Here's how the part is built. I have some questions about the finished solid (model axes, mm). A direction names the side the tool comes from. Round coordinates to 2 decimals unless told otherwise and drop trailing zeros. Loops run counter-clockwise (first coordinate to the right, second up) from the corner with the lowest first, then second, coordinate; pieces in that order, holes last. Notation, with made-up numbers: (20.25, -18.5) -> (41.25, -18.5) arc R13 ccw to (41.25, -5.5) -> close; hole circle Ø1 at (89, 88.5). An arc over 180 degrees is marked (long way). One line per item, written item: value. Start each with the question number.
```python
from build123d import *

# Parameters (mm, degrees)
SKETCH1_W           = 5.08
SKETCH1_H           = 203.2
BOSS_EXTRUDE1_DEPTH = 152.4
SKETCH2_W           = 88.9
SKETCH2_H           = 50.8
CUT_EXTRUDE1_DEPTH  = 5.08
SKETCH3_W           = 5.08
SKETCH3_H           = 10.16
CUT_EXTRUDE2_DEPTH  = 5.08
SKETCH5_W           = 5.08
SKETCH5_H           = 25.4
BOSS_EXTRUDE2_DEPTH = 5.08
SKETCH6_W           = 25.4
SKETCH6_H           = 5.08
SKETCH6_W_2         = 5.08
SKETCH6_H_2         = 25.4
CUT_EXTRUDE3_DEPTH  = 5.08


with BuildPart() as part:
    # Sketch1 → Boss-Extrude1 (new body)
    with BuildSketch(Plane.XY):
        with Locations((-99.06, 0)):
            Rectangle(SKETCH1_W, SKETCH1_H)
    extrude(amount=BOSS_EXTRUDE1_DEPTH)

    # Sketch2 → Cut-Extrude1 (cut)
    with BuildSketch(Plane.ZY.offset(101.6)):
        with Locations((107.95, -76.2)):
            Rectangle(SKETCH2_W, SKETCH2_H)
    extrude(amount=-CUT_EXTRUDE1_DEPTH, mode=Mode.SUBTRACT)

    # Sketch3 → Cut-Extrude2 (cut)
    with BuildSketch(Plane.XZ.offset(101.6)):
        with Locations((-99.06, 46.99)):
            Rectangle(SKETCH3_W, SKETCH3_H)
        with Locations((-99.06, 16.51)):
            Rectangle(SKETCH3_W, SKETCH3_H)
    extrude(amount=-CUT_EXTRUDE2_DEPTH, mode=Mode.SUBTRACT)

    # Sketch5 → Boss-Extrude2 (add)
    with BuildSketch(Plane(origin=(0, 0, 0), x_dir=(-1, 0, 0), z_dir=(0, 0, -1))):
        with Locations((99.06, -44.45)):
            Rectangle(SKETCH5_W, SKETCH5_H)
        with Locations((99.06, 63.5)):
            Rectangle(SKETCH5_W, SKETCH5_H)
    extrude(amount=BOSS_EXTRUDE2_DEPTH)

    # Sketch6 → Cut-Extrude3 (cut)
    with BuildSketch(Plane(origin=(-96.52, 0, 0), x_dir=(0, 0, -1), z_dir=(1, 0, 0))):
        with Locations((-114.3, 99.06)):
            Rectangle(SKETCH6_W, SKETCH6_H)
        with Locations((-33.02, 99.06)):
            Rectangle(SKETCH6_W, SKETCH6_H)
        with Locations((-149.86, 66.04)):
            Rectangle(SKETCH6_W_2, SKETCH6_H_2)
        with Locations((-149.86, -16.51)):
            Rectangle(SKETCH6_W_2, SKETCH6_H_2)
    extrude(amount=-CUT_EXTRUDE3_DEPTH, mode=Mode.SUBTRACT)


solid = part.part
```
Q1. Will these pins go through, and if not, where does the flat tip stop? P1, Ø1.5, axis at x = -99.5, z = 46.5, coming from the -Y side; P2, Ø2.5, axis at x = -100, y = -99.5, coming from the +Z side; P3, Ø2.5, axis at x = -99.5, z = 116, coming from the +Y side.
Q2. If we mould it in two halves opening along Z, with no side actions, what happens to faces 1 (the flat face through (-101.6, -1, 73)), 2 (the flat face through (-99, 66, 147.32)), 3 (the flat face through (-99, -99, 11.43))? For each: released by +Z, released by -Z, zero draft, split by the parting line, or undercut.
Q3. I want a section at B-B on z = 28. Please give me the cut outline in (x, y).
Q4. Which directions (+Z, -Z, +X, -X, +Y, -Y) give clear straight access to the entire face, cutting with the end or side of a thin tool? Please do faces 4 (the flat face through (-99, 78.74, 150)), 5 (the flat face through (-99, 99, 101.6)), 6 (the flat face through (-99, -99, 21.59)), 7 (the flat face through (-99, -31.75, -3)), 8 (the flat face through (-99, 76.2, -3)).
Q5. I want a section at A-A on y = 62.5. Please give me the cut outline in (x, z), plus the area to 3 significant figures.
Q6. If I drill on line 1 along Y through (x, z) = (-99.55, 77); line 2 along Z through (x, y) = (-97.1, -18.5); line 3 along Y through (x, z) = (-99.2, 22), over which ranges is the centre line in solid material (lowest first)?
Answers below:
1. P1: stops at y = -96.52
1. P2: stops at z = 63.5
1. P3: stops at y = 96.52
2. face 1: zero draft
2. face 2: released by +Z
2. face 3: undercut
3. outline: (-101.6, -101.6) -> (-96.52, -101.6) -> (-96.52, 96.52) -> (-101.6, 96.52) -> close
4. face 4: +Z, +X, -X
4. face 5: +X, -X, +Y
4. face 6: +X, -X, -Y
4. face 7: -Z, +X, -X
4. face 8: -Z, +X, -X, +Y
5. outline: (-101.6, -5.08) -> (-96.52, -5.08) -> (-96.52, 147.32) -> (-101.6, 147.32) -> close
5. area: 774 mm^2
6. line 1: y = -50.8 to 101.6
6. line 2: z = 0 to 147.32
6. line 3: y = -101.6 to 96.52
